Verification items for this drawing (mm, ordinates from the low corner). Round coordinates to 2 decimals unless told otherwise and drop trailing zeros. Order: outer loops, then holes, each group sorted by start corner. A loop starts at its lowest first (then second) coordinate and runs counter-clockwise, first axis right, second up. Notation, with made-up numbers: (33.5, -22.5) -> (73.5, -22.5) arc R17 ccw to (73.5, -9.5) -> close; hole circle Ø6 at (25, 5.5). An arc over 180 degrees is marked (long way). Answer in a Markdown table with one row per item. Add a question column.
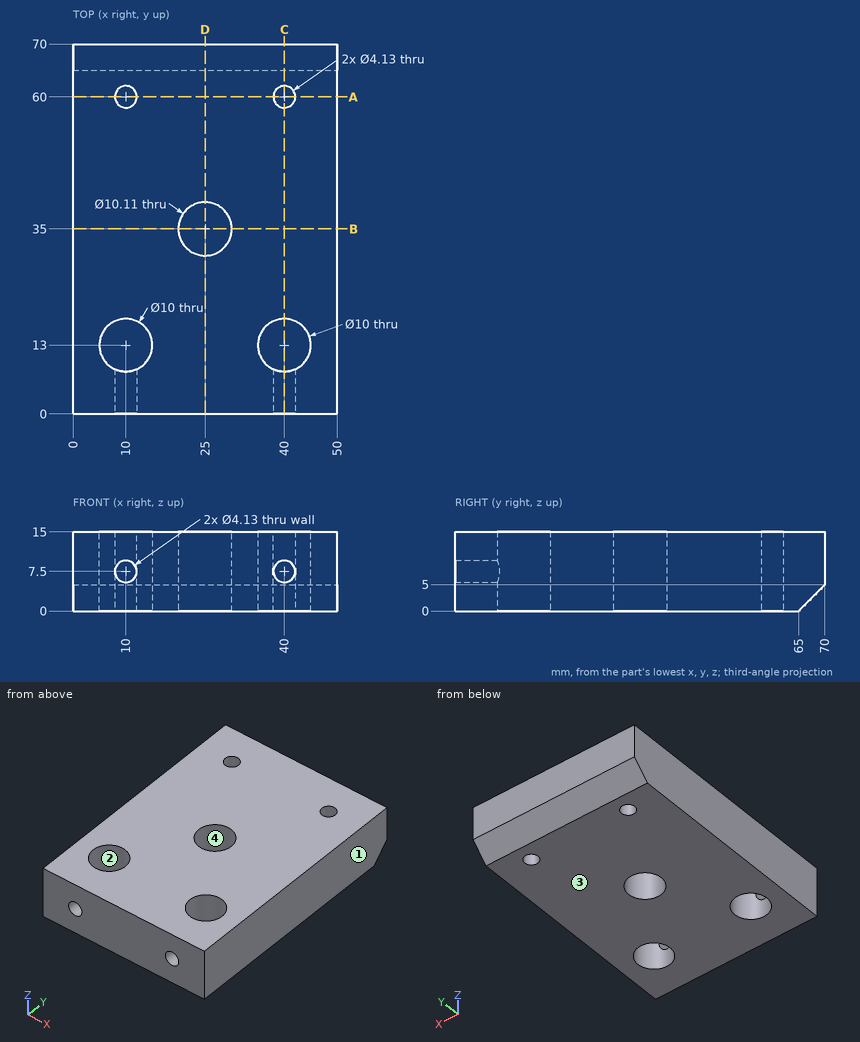
1) Cross-section at B-B, the plane y = 35. Record the boundary of the cut face in (x, z) (3 decimals), and give its area (3 significant figures).
2) Depth check by flat-ended pin: P1, Ø8, axis at x = 10, y = 13, coming from the -Z side (3 decimals); P2, Ø6, axis at x = 41.5, z = 7, coming from the -Y side. Enter the tip coordinate at first touch or a pass-through.
3) Cross-section at A-A, the plane y = 60. Record the boundary of the cut face in (x, z) (3 decimals), and give its area (3 significant figures).
4) Draft check along X on the marked faces 1, 2, 3 and 4. Enter one of: +X half, -X half, draft (parallel to the pull), parting line (faces both ways), or undercut.
5) Cross-section at C-C, the plane x = 40. Record the boundary of the cut face in (y, z) (3 decimals).
6) Cross-section at D-D, the plane x = 25. Record the boundary of the cut face in (y, z) (3 decimals), and give its area (3 significant figures).
7) Thickness scan on L1, parallel to Y at x = 10, z = 11.25 (3 decimals); L2, parallel to Y at x = 10, z = 3.25 (3 decimals); L3, parallel to X at y = 9, z = 4.5. Record the ranges inside material, lowest first. Write a range as [from, to].
Results below:
| question | item | result |
|---|---|---|
| 1 | outline | (0, 0) -> (19.945, 0) -> (19.945, 15) -> (0, 15) -> close; (30.055, 0) -> (50, 0) -> (50, 15) -> (30.055, 15) -> close |
| 1 | area | 598 mm² |
| 2 | P1 | through |
| 2 | P2 | y = 0 |
| 3 | outline | (0, 0) -> (7.935, 0) -> (7.935, 15) -> (0, 15) -> close; (12.065, 0) -> (37.935, 0) -> (37.935, 15) -> (12.065, 15) -> close; (42.065, 0) -> (50, 0) -> (50, 15) -> (42.065, 15) -> close |
| 3 | area | 626 mm² |
| 4 | face 1 | +X half |
| 4 | face 2 | undercut |
| 4 | face 3 | draft |
| 4 | face 4 | undercut |
| 5 | outline | (0, 0) -> (8, 0) -> (8, 5.435) -> (0, 5.435) -> close; (0, 9.565) -> (8, 9.565) -> (8, 15) -> (0, 15) -> close; (18, 0) -> (57.935, 0) -> (57.935, 15) -> (18, 15) -> close; (62.065, 0) -> (65, 0) -> (70, 5) -> (70, 15) -> (62.065, 15) -> close |
| 6 | outline | (0, 0) -> (29.945, 0) -> (29.945, 15) -> (0, 15) -> close; (40.055, 0) -> (65, 0) -> (70, 5) -> (70, 15) -> (40.055, 15) -> close |
| 6 | area | 886 mm² |
| 7 | L1 | [0, 8], [18, 57.935], [62.065, 70] |
| 7 | L2 | [0, 8], [18, 57.935], [62.065, 68.25] |
| 7 | L3 | [0, 7], [13, 37], [43, 50] |
